The listing builds one solid part. Answer for the finished solid, in the listing's coordinates (mm). A direction names the side the tool comes from. Coordinates: 2 decimals unless noted, no trailing zeros. Order: outer loops, then holes, each group sorted by start corner. A loop starts at its lowest first (then second) coordinate and runs counter-clockwise, first axis right, second up. Notation, with made-up numbers: (-4, -7) - (24, -7) arc R21 ccw to (24, 3) - close; hole circle Ø5 at (45, 42.5). An arc over 180 degrees is marked (long way). Use one line per item in the form item = value. Start each with the question number.
Item 1: Section D-D, the plane z = 111 is taken. Write down the section's boundary in (x, y).
Item 2: A tool of negligible diameter and unlimited length cuts with its end or side. For faces 5 (the flat face through (58, -46, 316)), 6 (the flat face through (60, -45, 156)), from which of +Z, -Z, +X, -X, +Y, -Y can it reach the whole face along a straight path? Write none if from no direction.
Item 3: Section C-C, the plane z = 7.5 is taken. Write down the section's boundary in (x, y), and give its area (3 significant figures).
Item 4: Section A-A, the plane x = 106.5 is taken. Write down the section's boundary in (y, z), and give its area (3 significant figures).
Item 5: Section B-B, the plane y = -37.5 is taken. Write down the section's boundary in (x, z), and give its area (3 significant figures).
Item 6: Each of these flat-tipped pins is pushed along its axis until it touches: pin 1 Ø5 at (x, z) = (36.5, 7.5) entering from +Y; pin 2 Ø7 at (x, z) = (106.5, 308.5) entering from +Y; pin 3 Ø22.5 at (y, z) = (-17.5, 132) entering from +X. Where does it stop, or does it pass through?
Item 7: Consider line 1 along Y through (x, z) = (1.05, 308.5); line 2 along X through (y, z) = (-45.8, 308.5); line 3 along Y through (x, z) = (46, 294). Determine where each line is inside the solid, lowest interval first. Write a range as [from, to].
Item 8: The mould has two halves that part along X. Classify faces 1 (the cylindrical face through (105.35, -45.76, 305.73)), 2 (the flat face through (0, -23, 156)), 3 (the cylindrical face through (103.838, -45.76, 6.116)), 4 (the flat face through (57, -46.5, 156)): released by +X, released by -X, zero draft, split by the parting line, or undercut.
from build123d import *

# Parameters (mm, degrees)
BOSS_EXTRUDE1_DEPTH = 316
CUT_EXTRUDE1_REACH  = 341.986
SKETCH2_R           = 3
CUT_EXTRUDE2_REACH  = 341.986
SKETCH3_R           = 3


with BuildPart() as part:
    # Sketch1 → Boss-Extrude1 (new body)
    with BuildSketch(Plane.XY):
        Polygon((0, 0), (0, -46.5), (116.5, -46.5), (116.5, -45), (1.5, -45), (1.5, 0), align=None)
    extrude(amount=BOSS_EXTRUDE1_DEPTH)

    # Sketch2 → Cut-Extrude1 (cut, up to next)
    with BuildSketch(Plane.ZY, mode=Mode.PRIVATE) as cut_extrude1_sk1:
        with Locations(Location((7.5, -7.5, 0), (0, 0, 270))):
            Circle(SKETCH2_R)
    cut_extrude1_tool1 = extrude(cut_extrude1_sk1.sketch, amount=-CUT_EXTRUDE1_REACH, mode=Mode.PRIVATE) & part.part
    # Sketch2 → Cut-Extrude1 (cut, up to next)
    with BuildSketch(Plane.ZY, mode=Mode.PRIVATE) as cut_extrude1_sk2:
        with Locations(Location((7.5, -37.5, 0), (0, 0, 270))):
            Circle(SKETCH2_R)
    cut_extrude1_tool2 = extrude(cut_extrude1_sk2.sketch, amount=-CUT_EXTRUDE1_REACH, mode=Mode.PRIVATE) & part.part
    # Sketch2 → Cut-Extrude1 (cut, up to next)
    with BuildSketch(Plane.ZY, mode=Mode.PRIVATE) as cut_extrude1_sk3:
        with Locations(Location((308.5, -37.5, 0), (0, 0, 270))):
            Circle(SKETCH2_R)
    cut_extrude1_tool3 = extrude(cut_extrude1_sk3.sketch, amount=-CUT_EXTRUDE1_REACH, mode=Mode.PRIVATE) & part.part
    # Sketch2 → Cut-Extrude1 (cut, up to next)
    with BuildSketch(Plane.ZY, mode=Mode.PRIVATE) as cut_extrude1_sk4:
        with Locations(Location((308.5, -7.5, 0), (0, 0, 270))):
            Circle(SKETCH2_R)
    cut_extrude1_tool4 = extrude(cut_extrude1_sk4.sketch, amount=-CUT_EXTRUDE1_REACH, mode=Mode.PRIVATE) & part.part
    add(cut_extrude1_tool1.solids().sort_by_distance((0, -7.5, 7.5))[0], mode=Mode.SUBTRACT)
    add(cut_extrude1_tool2.solids().sort_by_distance((0, -37.5, 7.5))[0], mode=Mode.SUBTRACT)
    add(cut_extrude1_tool3.solids().sort_by_distance((0, -37.5, 308.5))[0], mode=Mode.SUBTRACT)
    add(cut_extrude1_tool4.solids().sort_by_distance((0, -7.5, 308.5))[0], mode=Mode.SUBTRACT)

    # Sketch3 → Cut-Extrude2 (cut, up to next)
    with BuildSketch(Plane.XZ.offset(46.5), mode=Mode.PRIVATE) as cut_extrude2_sk1:
        with Locations(Location((106.5, 308.5, 0), (0, 0, 270))):
            Circle(SKETCH3_R)
    cut_extrude2_tool1 = extrude(cut_extrude2_sk1.sketch, amount=-CUT_EXTRUDE2_REACH, mode=Mode.PRIVATE) & part.part
    # Sketch3 → Cut-Extrude2 (cut, up to next)
    with BuildSketch(Plane.XZ.offset(46.5), mode=Mode.PRIVATE) as cut_extrude2_sk2:
        with Locations(Location((36.5, 308.5, 0), (0, 0, 270))):
            Circle(SKETCH3_R)
    cut_extrude2_tool2 = extrude(cut_extrude2_sk2.sketch, amount=-CUT_EXTRUDE2_REACH, mode=Mode.PRIVATE) & part.part
    # Sketch3 → Cut-Extrude2 (cut, up to next)
    with BuildSketch(Plane.XZ.offset(46.5), mode=Mode.PRIVATE) as cut_extrude2_sk3:
        with Locations(Location((106.5, 7.5, 0), (0, 0, 270))):
            Circle(SKETCH3_R)
    cut_extrude2_tool3 = extrude(cut_extrude2_sk3.sketch, amount=-CUT_EXTRUDE2_REACH, mode=Mode.PRIVATE) & part.part
    # Sketch3 → Cut-Extrude2 (cut, up to next)
    with BuildSketch(Plane.XZ.offset(46.5), mode=Mode.PRIVATE) as cut_extrude2_sk4:
        with Locations(Location((36.5, 7.5, 0), (0, 0, 270))):
            Circle(SKETCH3_R)
    cut_extrude2_tool4 = extrude(cut_extrude2_sk4.sketch, amount=-CUT_EXTRUDE2_REACH, mode=Mode.PRIVATE) & part.part
    add(cut_extrude2_tool1.solids().sort_by_distance((106.5, -46.5, 308.5))[0], mode=Mode.SUBTRACT)
    add(cut_extrude2_tool2.solids().sort_by_distance((36.5, -46.5, 308.5))[0], mode=Mode.SUBTRACT)
    add(cut_extrude2_tool3.solids().sort_by_distance((106.5, -46.5, 7.5))[0], mode=Mode.SUBTRACT)
    add(cut_extrude2_tool4.solids().sort_by_distance((36.5, -46.5, 7.5))[0], mode=Mode.SUBTRACT)


solid = part.part
Response:
q1.outline = (0, -46.5) - (116.5, -46.5) - (116.5, -45) - (1.5, -45) - (1.5, 0) - (0, 0) - close
q2.face_5 = +Z, +X, -X, +Y, -Y
q2.face_6 = +Z, -Z, +X, +Y
q3.outline = (0, -46.5) - (33.5, -46.5) - (33.5, -45) - (1.5, -45) - (1.5, -40.5) - (0, -40.5) - close; (0, -34.5) - (1.5, -34.5) - (1.5, -10.5) - (0, -10.5) - close; (0, -4.5) - (1.5, -4.5) - (1.5, 0) - (0, 0) - close; (39.5, -46.5) - (103.5, -46.5) - (103.5, -45) - (39.5, -45) - close; (109.5, -46.5) - (116.5, -46.5) - (116.5, -45) - (109.5, -45) - close
q3.area = 206 mm2
q4.outline = (-46.5, 0) - (-45, 0) - (-45, 4.5) - (-46.5, 4.5) - close; (-46.5, 10.5) - (-45, 10.5) - (-45, 305.5) - (-46.5, 305.5) - close; (-46.5, 311.5) - (-45, 311.5) - (-45, 316) - (-46.5, 316) - close
q4.area = 456 mm2
q5.outline = (0, 0) - (1.5, 0) - (1.5, 4.5) - (0, 4.5) - close; (0, 10.5) - (1.5, 10.5) - (1.5, 305.5) - (0, 305.5) - close; (0, 311.5) - (1.5, 311.5) - (1.5, 316) - (0, 316) - close
q5.area = 456 mm2
q6.pin_1 = through
q6.pin_2 = -45
q6.pin_3 = 1.5
q7.line_1 = [-46.5, -40.5], [-34.5, -10.5], [-4.5, 0]
q7.line_2 = [0, 33.5], [39.5, 103.5], [109.5, 116.5]
q7.line_3 = [-46.5, -45]
q8.face_1 = undercut
q8.face_2 = released by -X
q8.face_3 = undercut
q8.face_4 = zero draft
